```python
from build123d import *

# Parameters (mm, degrees)
EXTRUDE_THIN1_DEPTH     = 88.9
CUT_EXTRUDE1_DEPTH      = 1
CUT_EXTRUDE1_DEPTH_BACK = 39.1


with BuildPart() as part:
    # Sketch1 → Extrude-Thin1 (new body, symmetric)
    with BuildSketch(Plane(origin=(0, 0, 0), x_dir=(0, 0, -1), z_dir=(1, 0, 0))):
        with BuildLine():
            Line((-15.875, 19.05), (15.875, 19.05))
            ThreePointArc((15.875, 19.05), (18.12006403, 18.12006403), (19.05, 15.875))
            Line((19.05, 15.875), (19.05, -15.875))
            ThreePointArc((19.05, -15.875), (18.12006403, -18.12006403), (15.875, -19.05))
            Line((15.875, -19.05), (-15.875, -19.05))
            ThreePointArc((-15.875, -19.05), (-18.12006403, -18.12006403), (-19.05, -15.875))
            Line((-19.05, -15.875), (-19.05, 15.875))
            ThreePointArc((-19.05, 15.875), (-18.12006403, 18.12006403), (-15.875, 19.05))
        make_face()
        with BuildLine():
            Line((-15.875, 16.51), (15.875, 16.51))
            ThreePointArc((15.875, 16.51), (16.324012806, 16.324012806), (16.51, 15.875))
            Line((16.51, 15.875), (16.51, -15.875))
            ThreePointArc((16.51, -15.875), (16.324012806, -16.324012806), (15.875, -16.51))
            Line((15.875, -16.51), (-15.875, -16.51))
            ThreePointArc((-15.875, -16.51), (-16.324012806, -16.324012806), (-16.51, -15.875))
            Line((-16.51, -15.875), (-16.51, 15.875))
            ThreePointArc((-16.51, 15.875), (-16.324012806, 16.324012806), (-15.875, 16.51))
        make_face(mode=Mode.SUBTRACT)
    extrude(amount=EXTRUDE_THIN1_DEPTH, both=True)

    # Sketch2 → Cut-Extrude1 (cut, two sides)
    with BuildSketch(Plane.XY.offset(19.05)) as cut_extrude1_sk:
        Polygon((275.736327504, -342.660011936), (88.9, -19.05), (66.902954744, 19.05), (-119.93337276, 342.660011936), (527.286651112, 716.332666943), (922.956351375, 31.012643071), align=None)
    extrude(amount=CUT_EXTRUDE1_DEPTH, mode=Mode.SUBTRACT)
    extrude(cut_extrude1_sk.sketch, amount=-CUT_EXTRUDE1_DEPTH_BACK, mode=Mode.SUBTRACT)


solid = part.part
```
The model under review builds one solid part; all positions refer to its coordinate system, in mm. A direction names the side the tool comes from. Round coordinates to 2 decimals unless told otherwise and drop trailing zeros. Order: outer loops, then holes, each group sorted by start corner. A loop starts at its lowest first (then second) coordinate and runs counter-clockwise, first axis right, second up. Notation, with made-up numbers: (28, 0) -> (58, 0) arc R28 cw to (58, 18) -> close; hole circle Ø9 at (27, -35). An arc over 180 degrees is marked (long way). One line per item, written item: value. Start each with the question number.
Q1. Clearance check with a flat-ended pin moving along its axis: pin 1 Ø12 at (y, z) = (8, -4.5) entering from +X. State where the tip first meets the part, or that it passes through.
Q2. Take a section at D-D (x = 76). Write out the cut boundary in (y, z) (3 decimals).
Q3. Mouldability with a two-part tool opening along Y and no side actions: class faces 3 (the face through (1.24, -18.14, 18.1)), 4 (the face through (0, 0, 16.51)), 5 (the face through (-88.9, 0, -17)), 6 (the face through (0, 0, -16.51)) as released by +Y, released by -Y, zero draft, split by the parting line, or undercut.
Q4. Wall thickness on line 1 (Y direction, x = 36, z = -1.5): over which ranges is the line inside the solid? List them lowest first.
Q5. Machinability: for faces 1 (the face through (78.055, -0.267, -16.667)), 2 (the face through (1, -16.51, 0)), which of the approach directions +Z, -Z, +X, -X, +Y, -Y give a long, thin tool a straight path to every point of the face, cutting with its end or side? Answer none if there is none.
Q6. Take a section at A-A (z = -12). Write out the cut boundary in (x, y), and give its area (3 significant figures).
Q7. Take a section at B-B (x = 9). Write out the cut boundary in (y, z) (3 decimals).
Q8. Take a section at C-C (y = -12). Write out the cut boundary in (x, z), and give its area (3 significant figures).
Reported:
1. pin 1: passes through
2. outline: (-19.05, -15.875) arc R3.175 ccw to (-15.875, -19.05) -> (3.293, -19.05) -> (3.293, -16.51) -> (-15.875, -16.51) arc R0.635 cw to (-16.51, -15.875) -> (-16.51, 15.875) arc R0.635 cw to (-15.875, 16.51) -> (3.293, 16.51) -> (3.293, 19.05) -> (-15.875, 19.05) arc R3.175 ccw to (-19.05, 15.875) -> close
3. face 3: released by -Y
3. face 4: undercut
3. face 5: zero draft
3. face 6: undercut
4. line 1: y = -19.05 to -16.51, 16.51 to 19.05
5. face 1: +Z, -Z, +X, +Y
5. face 2: +X, -X
6. outline: (-88.9, -19.05) -> (88.9, -19.05) -> (87.43, -16.51) -> (-88.9, -16.51) -> close; (-88.9, 16.51) -> (68.37, 16.51) -> (66.9, 19.05) -> (-88.9, 19.05) -> close
6. area: 847 mm2
7. outline: (-19.05, -15.875) arc R3.175 ccw to (-15.875, -19.05) -> (15.875, -19.05) arc R3.175 ccw to (19.05, -15.875) -> (19.05, 15.875) arc R3.175 ccw to (15.875, 19.05) -> (-15.875, 19.05) arc R3.175 ccw to (-19.05, 15.875) -> close; hole (-16.51, -15.875) arc R0.635 ccw to (-15.875, -16.51) -> (15.875, -16.51) arc R0.635 ccw to (16.51, -15.875) -> (16.51, 15.875) arc R0.635 ccw to (15.875, 16.51) -> (-15.875, 16.51) arc R0.635 ccw to (-16.51, 15.875) -> close
8. outline: (-88.9, -19.05) -> (84.83, -19.05) -> (84.83, -16.51) -> (-88.9, -16.51) -> close; (-88.9, 16.51) -> (84.83, 16.51) -> (84.83, 19.05) -> (-88.9, 19.05) -> close
8. area: 883 mm2
